Autodesk Fusion 360 part; units mm, degrees
sketch "スケッチ1" plane through (0, 0, 0) normal (0, 0, 1) x (1, 0, 0)
  line L0 (0, 0) -> (14, 0)
  line L1 (14, 0) -> (14, 10)
  line L2 (14, 10) -> (0, 10)
  line L3 (0, 10) -> (0, 0)
  line L4 (21.8, 0) -> (38.8, 0)
  line L5 (38.8, 0) -> (38.8, 10)
  line L6 (38.8, 10) -> (21.8, 10)
  line L7 (21.8, 10) -> (21.8, 0)
  line L8 (0.5, 9.5) -> (0.5, 0.5)
  line L9 (0.5, 0.5) -> (13.5, 0.5)
  line L10 (13.5, 0.5) -> (13.5, 9.5)
  line L11 (13.5, 9.5) -> (0.5, 9.5)
  line L12 (22.3, 0.5) -> (38.3, 0.5)
  line L13 (38.3, 0.5) -> (38.3, 9.5)
  line L14 (38.3, 9.5) -> (22.3, 9.5)
  line L15 (22.3, 9.5) -> (22.3, 0.5)
  line L16 (0, 38) -> (14, 38)
  line L17 (14, 38) -> (14, 48)
  line L18 (14, 48) -> (0, 48)
  line L19 (0, 48) -> (0, 38)
  line L20 (0.5, 38.5) -> (13.5, 38.5)
  line L21 (13.5, 38.5) -> (13.5, 47.5)
  line L22 (13.5, 47.5) -> (0.5, 47.5)
  line L23 (0.5, 47.5) -> (0.5, 38.5)
  line L24 (-2, 50) -> (-2, -6.35)
  line L25 (-2, -6.35) -> (40.8, -6.35)
  line L26 (40.8, -6.35) -> (40.8, 9.0983)
  line L27 (40.8, 9.0983) -> (16, 50)
  line L28 (16, 50) -> (-2, 50)
  line L29 (17.95, 10) -> (19.45, 10)
  line L30 (19.45, 10) -> (19.45, 0)
  line L31 (17.95, 0) -> (17.95, 10)
  line L32 (17.2, 10) -> (17.2, 0)
  line L33 (20.2, 10) -> (20.2, 0)
  arc A0 (19.45, 10) -> (17.95, 10) centre (18.7, 10) ccw
  arc A1 (20.2, 10) -> (17.2, 10) centre (18.7, 10) ccw
  arc A2 (17.95, 0) -> (19.45, 0) centre (18.7, 0) ccw
  arc A3 (17.2, 0) -> (20.2, 0) centre (18.7, 0) ccw
  circle A4 centre (1.2, -6.35) radius 1.5
  circle A5 centre (37.6, -6.35) radius 1.5
  line L34 (-2, -6.35) -> (-2, -9.55)
  line L35 (-2, -9.55) -> (40.8, -9.55)
  line L36 (40.8, -9.55) -> (40.8, -6.35)
  line L37 (1.2, -7.85) -> (37.6, -7.85)
  line L38 (37.6, -4.85) -> (1.2, -4.85)
  line L39 (-2, -2) -> (40.8, -2)
  dimension "d1" = 14
  dimension "d2" = 10
  dimension "d3" = 17
  dimension "d4" = 10
  dimension "d5" = 7.8
  dimension "d6" = -0.5
  dimension "d7" = -0.5
  dimension "d8" = 14
  dimension "d9" = 10
  dimension "d10" = 28
  dimension "d11" = -0.5
  dimension "d12" = 2
  dimension "d13" = 2
  dimension "d14" = 2
  dimension "d15" = 14
  dimension "d16" = 6.35
  dimension "d17" = 2
  dimension "d39" = 1.5
  dimension "d40" = 3.95
  dimension "d41" = 0.75
  dimension "d42" = 0.75
  dimension "d45" = 3
  dimension "d46" = 3
  dimension "d47" = 3.2
  dimension "d48" = 3.2
  dimension "d49" = 3.2
  dimension "d50" = 2
extrude "押し出し1" add sketch "スケッチ1" against normal blind 45.2 contours L8 L9 L10 L11 | L12 L13 L14 L15 | L20 L21 L22 L23 makes body 1 at (4.8333, 38.5, -30.1333) makes body 2 at (9.1667, 9.5, -15.0667) makes body 3 at (32.9667, 9.5, -30.1333)
extrude "押し出し2" add sketch "スケッチ1" along normal blind 8 contours L0 L1 L2 L3 | L4 L5 L6 L7 | L8 L9 L10 L11 | L12 L13 L14 L15 | L16 L17 L18 L19 | L20 L21 L22 L23 | L24 L26 L27 L28 L39 bodies 1 2 3
fillet "フィレット1" radius 2.5 12 edges at (38.3, 9.5, -22.6) (38.3, 0.5, -22.6) (13.5, 9.5, -22.6) (13.5, 0.5, -22.6) (13.5, 38.5, -22.6) (13.5, 47.5, -22.6) (22.3, 0.5, -22.6) (22.3, 9.5, -22.6) (0.5, 38.5, -22.6) (0.5, 47.5, -22.6) (0.5, 9.5, -22.6) (0.5, 0.5, -22.6) on bodies 1
fillet "フィレット2" radius 2 24 edges at (1.2322, 8.7678, 0) (7, 9.5, 0) (12.7678, 8.7678, 0) (13.5, 5, 0) (12.7678, 1.2322, 0) (7, 0.5, 0) (1.2322, 1.2322, 0) (0.5, 5, 0) (23.0322, 8.7678, 0) (30.3, 9.5, 0) (37.5678, 8.7678, 0) (38.3, 5, 0) (37.5678, 1.2322, 0) (30.3, 0.5, 0) (23.0322, 1.2322, 0) (22.3, 5, 0) (12.7678, 46.7678, 0) (13.5, 43, 0) (12.7678, 39.2322, 0) (7, 38.5, 0) (1.2322, 39.2322, 0) (0.5, 43, 0) (1.2322, 46.7678, 0) (7, 47.5, 0) on bodies 1
sketch "スケッチ2" plane through (0, 0.5, 0) normal (0, -1, 0) x (1, 0, 0)
  line L0 (11, -2) -> (3, -2)
  line L1 (3, -2) -> (3, -45.2)
  line L2 (3, -45.2) -> (11, -45.2)
  line L3 (11, -45.2) -> (11, -2)
  line L4 (10, -35) -> (27, -35)
  line L5 (27, -35) -> (27, -46)
  line L6 (27, -46) -> (10, -46)
  line L7 (10, -46) -> (10, -35)
  dimension "d26" = 17
  dimension "d27" = 11
  dimension "d28" = 46
  dimension "d29" = 10
extrude "押し出し3" cut sketch "スケッチ2" against normal blind 10 contours L2 L3 L4 L5 L6 L7 | L2 L3 L4 L7 bodies 1
extrude "押し出し5" add sketch "スケッチ1" along normal blind 2.2 contours L24 L25 L26 A4 A5 L38 L39 | L25 A4 A5 L34 L35 L36 L37 | L32 L33 A1 A3 bodies 1
fillet "フィレット3" radius 2.2 1 edges at (19.4, -2, 2.2) on bodies 1
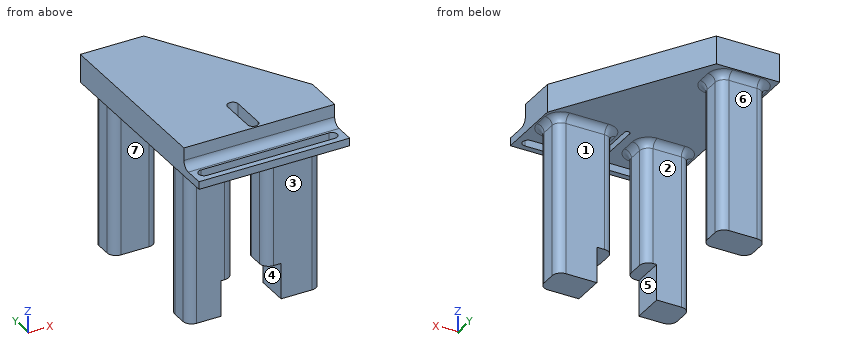
Geometry: final body of the model. Coordinates: model frame, mm. Face numbers are marked on the shaded views. A direction names the side the tool comes from. Coordinates: 2 decimals unless noted, no trailing zeros. Order: outer loops, then holes, each group sorted by start corner. A loop starts at its lowest first (then second) coordinate and runs counter-clockwise, first axis right, second up. Notation, with made-up numbers: (86.5, 32) -> (133.5, 32) arc R19 ccw to (133.5, 54) -> close; hole circle Ø3 at (50, -40). An arc over 180 degrees is marked (long way). Write each question's results on one line, items separated by ' | '. Start each with the question number.
1) Cut plane D-D, the plane x = 18.7. Output: boundary loops of the cut face in (y, z), and give its area (3 significant figures).
2) First-contact query: pin 1 (4 mm diameter, centred on x = 24, y = 7, fed in from -Z); pin 2 (3 mm diameter, centred on y = 5, z = -29, fed in from -X); pin 3 (3 mm diameter, centred on x = 28.5, z = -35.5, fed in from -Y); pin 4 (12 mm diameter, centred on x = 33.5, y = 43.5, fed in from -Z) (3 decimals). Flat tips, straight axial feed; report the tip coordinate or a pass-through.
3) Mould query, pull axis Y, two halves, no side actions, for the marked faces 5, 6 and 7. Classes: released by +Y, released by -Y, zero draft, split by the parting line, or undercut.
4) Set-up query: the marked faces 1, 2, 3 and 4. Return all of +Z, -Z, +X, -X, +Y, -Y with unobstructed straight access to the full face (end or side cutting, diameter ignored); none if empty.
5) Cut plane A-A, the plane y = -6.35. Output: boundary loops of the cut face in (x, z).
6) Cut plane C-C, the plane x = 33.5. Output: boundary loops of the cut face in (y, z).
7) Material intervals for line 1 along Y through (x, z) = (5, -9); line 2 along X through (y, z) = (6, -10); line 3 along Z through (x, y) = (11.5, 18), sorted ascending.
8) Cut plane B-B, the plane z = -32.5. Output: boundary loops of the cut face in (x, y).
Checks:
1) outline: (-9.55, 0) -> (-7.85, 0) -> (-7.85, 2.2) -> (-9.55, 2.2) -> close; (-4.85, 0) -> (-0.75, 0) -> (-0.75, 2.2) -> (-1.5, 2.2) -> (-1.5, 8) -> (-2, 8) -> (-2, 4.4) arc R2.2 cw to (-4.2, 2.2) -> (-4.85, 2.2) -> close; (10.75, 0) -> (45.55, 0) -> (45.55, 8) -> (11.5, 8) -> (11.5, 2.2) -> (10.75, 2.2) -> close | area: 291 mm^2
2) pin 1: z = -35 | pin 2: x = 0.5 | pin 3: y = 0.5 | pin 4: through
3) face 5: zero draft | face 6: released by +Y | face 7: undercut
4) face 1: -Z, +X, -X, +Y | face 2: -Z, +X, -X | face 3: -Z, +X, -X, -Y | face 4: -Z, +Y, -Y
5) outline: (-2, 0) -> (-0.3, 0) -> (-0.3, 2.2) -> (-2, 2.2) -> close; (39.1, 0) -> (40.8, 0) -> (40.8, 2.2) -> (39.1, 2.2) -> close
6) outline: (-9.55, 0) -> (-7.85, 0) -> (-7.85, 2.2) -> (-9.55, 2.2) -> close; (-4.85, 0) -> (-1.5, 0) arc R2 cw to (0.5, -2) -> (0.5, -45.2) -> (9.5, -45.2) -> (9.5, -2) arc R2 cw to (11.5, 0) -> (21.14, 0) -> (21.14, 8) -> (-2, 8) -> (-2, 4.4) arc R2.2 cw to (-4.2, 2.2) -> (-4.85, 2.2) -> close
7) line 1: 0.5 to 9.5, 38.5 to 47.5 | line 2: 0.5 to 13.5, 22.3 to 38.3 | line 3: 0 to 8
8) outline: (0.5, 3) arc R2.5 ccw to (3, 0.5) -> (11, 0.5) arc R2.5 ccw to (13.5, 3) -> (13.5, 7) arc R2.5 ccw to (11, 9.5) -> (3, 9.5) arc R2.5 ccw to (0.5, 7) -> close; (0.5, 41) arc R2.5 ccw to (3, 38.5) -> (11, 38.5) arc R2.5 ccw to (13.5, 41) -> (13.5, 45) arc R2.5 ccw to (11, 47.5) -> (3, 47.5) arc R2.5 ccw to (0.5, 45) -> close; (22.3, 3) arc R2.5 ccw to (24.8, 0.5) -> (35.8, 0.5) arc R2.5 ccw to (38.3, 3) -> (38.3, 7) arc R2.5 ccw to (35.8, 9.5) -> (24.8, 9.5) arc R2.5 ccw to (22.3, 7) -> close
